Solid Edge part; units mm, degrees
sketch "Sketch1" plane through (0, 0, 0) normal (0, -1, 0) x (1, 0, 0)
  line L0 (35, 17.5) -> (-35, 17.5)
  line L1 (-35, 17.5) -> (-35, -17.5)
  line L2 (-35, -17.5) -> (35, -17.5)
  line L3 (35, -17.5) -> (35, 17.5)
extrude "Protrusion1" add sketch "Sketch1" against normal blind 5
sketch "Sketch2" plane through (0, 0, 0) normal (0, -1, 0) x (1, 0, 0)
  circle A0 centre (17.5852, 0) radius 2.5
extrude "ExtrudedCutout_1" cut sketch "Sketch2" against normal blind 7
sketch "Sketch3" plane through (0, 0, 0) normal (0, -1, 0) x (1, 0, 0)
  circle A0 centre (-17.5, 0) radius 2.5
extrude "ExtrudedCutout_2" cut sketch "Sketch3" against normal blind 7
sketch "Sketch4" plane through (0, 5, 0) normal (0, 1, 0) x (-1, 0, 0)
  circle A0 centre (-31.25, -14.5) radius 1.5
extrude "ExtrudedCutout_10" cut sketch "Sketch4" against normal blind 7
sketch "Sketch5" plane through (0, 5, 0) normal (0, 1, 0) x (-1, 0, 0)
  circle A0 centre (31.25, -14.5) radius 1.5
extrude "ExtrudedCutout_11" cut sketch "Sketch5" against normal blind 7
shell "Thinwall_4" thickness 4 removed faces 1 at (-22.6333, 5, 12.0167)
sketch "Sketch6" plane through (0, 2.5, -17.5) normal (0, 0, -1) x (-1, 0, 0)
  line L0 (-6.5, 1.5) -> (-28.5, 1.5)
  line L1 (-28.5, 1.5) -> (-28.5, -1.5)
  line L2 (-28.5, -1.5) -> (-6.5, -1.5)
  line L3 (-6.5, -1.5) -> (-6.5, 1.5)
extrude "ExtrudedCutout_13" cut sketch "Sketch6" against normal blind 3.9
sketch "Sketch7" plane through (0, 2.5, -17.5) normal (0, 0, -1) x (-1, 0, 0)
  line L0 (2.5, 1.5) -> (-2.5, 1.5)
  line L1 (-2.5, 1.5) -> (-2.5, -1.5)
  line L2 (-2.5, -1.5) -> (2.5, -1.5)
  line L3 (2.5, -1.5) -> (2.5, 1.5)
extrude "ExtrudedCutout_14" cut sketch "Sketch7" against normal blind 3.9
sketch "Sketch8" plane through (0, 2.5, -17.5) normal (0, 0, -1) x (-1, 0, 0)
  line L0 (28.5, 1.5) -> (6.5, 1.5)
  line L1 (6.5, 1.5) -> (6.5, -1.5)
  line L2 (6.5, -1.5) -> (28.5, -1.5)
  line L3 (28.5, -1.5) -> (28.5, 1.5)
extrude "ExtrudedCutout_15" cut sketch "Sketch8" against normal blind 3.9
Geometry check sheet. Reference: the model listing, model coordinates, mm. A direction names the side the tool comes from. Give positions to 0.01 mm unless a question says otherwise; leave off trailing zeros. Loops run counter-clockwise (first coordinate to the right, second up) from the corner with the lowest first, then second, coordinate; pieces in that order, holes last. Notation, with made-up numbers: M 38,20.25 L 86,20.25 A22 cw 86,42.25 Z; hole C -20,41 d7. An arc over 180 degrees is marked long. Write item = value, one per line. Start each with the question number.
1. Section check D-D, the plane z = 0. Enter the section's corners in (x, y).
2. Section check C-C, the plane x = -9.5. Enter the section's corners in (y, z), plus the area to 3 significant figures.
3. Section check A-A, the plane z = -14.5. Enter the section's corners in (x, y), plus the area to 3 significant figures.
4. Tool access check on faces 1 (the face through (-35, 2, 0)), 2 (the face through (-23.994, 4.493, 0.286)), 3 (the face through (0, 1, -16)). Record the directions out of +Z, -Z, +X, -X, +Y, -Y that give a thin tool (end or side, any length) a straight path to the whole face; none if there is none.
5. Thickness scan on probe 1 along Z at (x, y) = (-31.25, 3.9); probe 2 along X at (y, z) = (4.8, 7.5); probe 3 along Z at (x, y) = (8, 4.6). Record the ranges inside material, lowest first.
6. Section check B-B, the plane y = 3. Enter the section's corners in (x, z), plus the area to 3 significant figures.
7. Draft check along Z on faces 4 (the face through (6.5, 2, -16)), 5 (the face through (-0.5, 0.8, -17.5)), 6 (the face through (-27.7, 4.5, -10.3)). Enter one of: +Z half, -Z half, draft (parallel to the pull), parting line (faces both ways), or undercut.
Values follow:
q1.outline = M -35,0 L -20,0 L -20,5 L -24,5 L -24,4 L -31,4 L -31,5 L -35,5 Z; M -15,0 L 15.09,0 L 15.09,5 L 11.09,5 L 11.09,4 L -11,4 L -11,5 L -15,5 Z; M 20.09,0 L 35,0 L 35,5 L 31,5 L 31,4 L 24.09,4 L 24.09,5 L 20.09,5 Z
q2.outline = M 0,-17.5 L 1,-17.5 L 1,-13.6 L 4,-13.6 L 4,-17.5 L 5,-17.5 L 5,-13.5 L 4,-13.5 L 4,13.5 L 5,13.5 L 5,17.5 L 0,17.5 Z
q2.area = 136 mm^2
q3.outline = M -35,0 L -32.75,0 L -32.75,5 L -35,5 Z; M -29.75,0 L 29.75,0 L 29.75,5 L -29.75,5 Z; M 32.75,0 L 35,0 L 35,5 L 32.75,5 Z; hole M -28.5,1 L -6.5,1 L -6.5,4 L -28.5,4 Z; hole M -2.5,1 L 2.5,1 L 2.5,4 L -2.5,4 Z; hole M 6.5,1 L 28.5,1 L 28.5,4 L 6.5,4 Z
q3.area = 173 mm^2
q4.face_1 = +Z, -Z, -X, +Y, -Y
q4.face_2 = +Y
q4.face_3 = -Z
q5.probe_1 = -17.5 to -16, -13 to 17.5
q5.probe_2 = -35 to -31, 31 to 35
q5.probe_3 = -17.5 to -13.5, 13.5 to 17.5
q6.outline = M -35,-17.5 L -28.5,-17.5 L -28.5,-13.6 L -6.5,-13.6 L -6.5,-17.5 L -2.5,-17.5 L -2.5,-13.6 L 2.5,-13.6 L 2.5,-17.5 L 6.5,-17.5 L 6.5,-13.6 L 28.5,-13.6 L 28.5,-17.5 L 35,-17.5 L 35,17.5 L -35,17.5 Z; hole C -31.25,-14.5 d3; hole C -17.5,0 d5; hole C 17.59,0 d5; hole C 31.25,-14.5 d3
q6.area = 2,210 mm^2
q7.face_4 = draft
q7.face_5 = -Z half
q7.face_6 = undercut
